Input: dimensioned drawing with shaded views. Units: mm. Origin: part minimum x, y, z. Round coordinates to 2 decimals unless told otherwise and drop trailing zeros. Write each loop counter-clockwise with the first axis right and the second up, starting at its lowest first coordinate (ties: lowest second). Pieces come first, ordered by that corner, then holes. Notation, with made-up numbers: M 79.5,75 L 133.5,75 A37 cw 133.5,114 Z; hole C 70.5,71 d3. An arc over 180 degrees is marked long. Use one line per item in the form item = value. Start each with the question number.
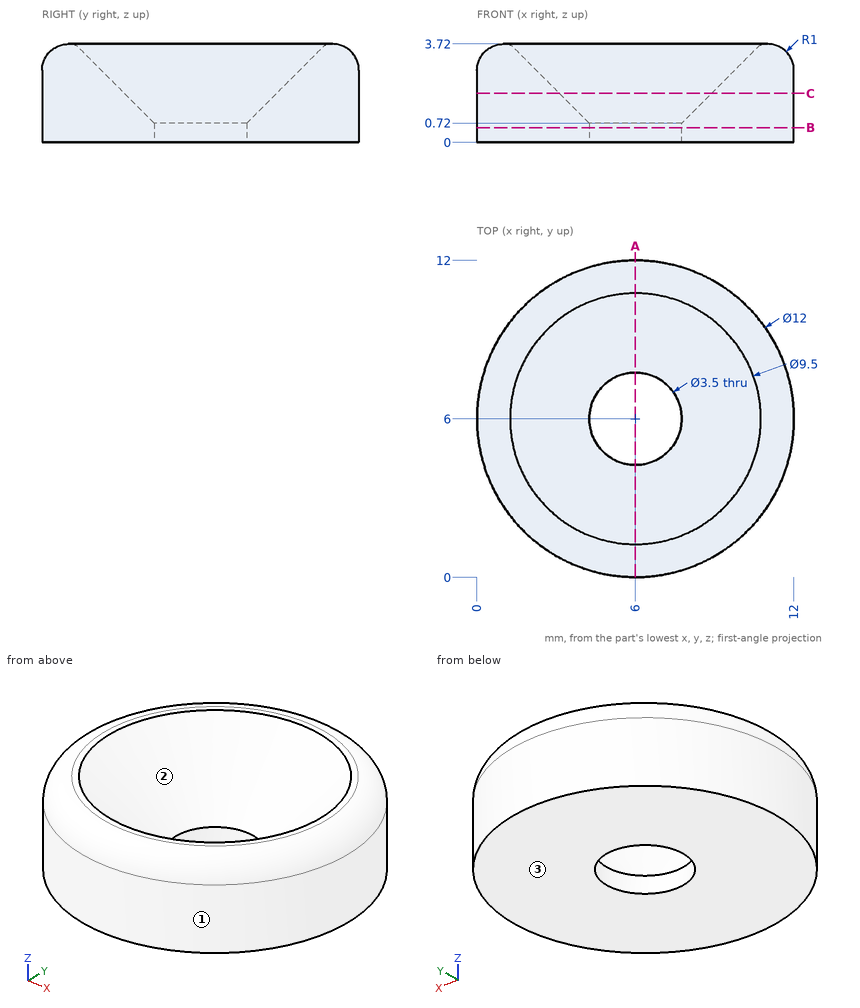
1. Section query B-B (z = 0.55). Return loops of the section in (x, y), then the cut area to 3 significant figures.
2. Ray query, probe 1 along X at (y, z) = (6, 0.25); probe 2 along Y at (x, z) = (3.5, 1.95). Return the intervals inside material, ascending.
3. Contact query for flat-ended pins moving along their axis: pin 1 (4 mm diameter, centred on x = 1.5, y = 6.5, fed in from +Z); pin 2 (1.5 mm diameter, centred on x = 7, y = 6.5, fed in from +Z). Output: stop coordinate, or through.
4. Section query A-A (x = 6). Return loops of the section in (y, z).
5. Section query C-C (z = 1.85). Return loops of the section in (x, y).
6. Pull-direction query (X, two-part tool) for the marked faces 1, 2 and 3; classes: released by +X, released by -X, zero draft, split by the parting line, or undercut.
Checks:
q1.outline = C 6,6 d12; hole C 6,6 d3.5
q1.area = 103 mm^2
q2.probe_1 = 0 to 4.25, 7.75 to 12
q2.probe_2 = 0.55 to 4.38, 7.62 to 11.45
q3.pin_1 = 3.72
q3.pin_2 = 0.84
q4.outline = M 0,0 L 4.25,0 L 4.25,0.72 L 1.25,3.72 L 1,3.72 A1 ccw 0,2.72 Z; M 7.75,0 L 12,0 L 12,2.72 A1 ccw 11,3.72 L 10.75,3.72 L 7.75,0.72 Z
q5.outline = C 6,6 d12; hole C 6,6 d5.76
q6.face_1 = split by the parting line
q6.face_2 = undercut
q6.face_3 = zero draft
